```python
from build123d import *

# Parameters (mm, degrees)
F1_DEPTH = 25.4
F2_R     = 6.35
F3_DEPTH = 25.401
F4_DEPTH = 19.05
F5_R     = 6.35
F6_DEPTH = 6.351


with BuildPart() as f1:
    # F0 (on Top) → F1 (new body)
    with BuildSketch(Plane.XY):
        with BuildLine():
            ThreePointArc((-11.9960894898, 7.8287454173), (-22.8140252531, 16.2307401146), (-25.7390544228, 29.6122741608))
            ThreePointArc((-25.7390544228, 29.6122741608), (-33.3767507176, 24.6782589704), (-41.673253936, 28.3994073062))
            ThreePointArc((-41.673253936, 28.3994073062), (-43.3440087931, 16.5245060033), (-51.6016386333, 7.8287454173))
            ThreePointArc((-51.6016386333, 7.8287454173), (-44.8664465425, 5.0389375081), (-42.0766386333, -1.6962545827))
            ThreePointArc((-42.0766386333, -1.6962545827), (-43.013362785, -5.8153737791), (-45.6392933218, -9.1243137765))
            ThreePointArc((-45.6392933218, -9.1243137765), (-31.7988640615, -7.20255554), (-17.9584348012, -9.1243137765))
            ThreePointArc((-17.9584348012, -9.1243137765), (-20.9815746971, 1.463916392), (-11.9960894898, 7.8287454173))
        make_face()
        with BuildLine():
            ThreePointArc((-42.0766386333, -1.6962545827), (-44.8664465425, 5.0389375081), (-51.6016386333, 7.8287454173))
            ThreePointArc((-51.6016386333, 7.8287454173), (-61.1266386333, -1.6962545827), (-51.6016386333, -11.2212545827))
            ThreePointArc((-51.6016386333, -11.2212545827), (-48.6531092599, -10.0799677677), (-45.6392933218, -9.1243137765))
            ThreePointArc((-45.6392933218, -9.1243137765), (-43.013362785, -5.8153737791), (-42.0766386333, -1.6962545827))
        make_face()
        with BuildLine():
            ThreePointArc((-2.4710894898, -1.6962545827), (-5.260897399, 5.0389375081), (-11.9960894898, 7.8287454173))
            ThreePointArc((-11.9960894898, 7.8287454173), (-20.9815746971, 1.463916392), (-17.9584348012, -9.1243137765))
            ThreePointArc((-17.9584348012, -9.1243137765), (-14.9446188632, -10.0799677677), (-11.9960894898, -11.2212545827))
            ThreePointArc((-11.9960894898, -11.2212545827), (-5.260897399, -8.4314466735), (-2.4710894898, -1.6962545827))
        make_face()
        with BuildLine():
            ThreePointArc((-25.7390544228, 29.6122741608), (-25.2909601874, 31.9282439717), (-24.5746759409, 34.175785181))
            ThreePointArc((-24.5746759409, 34.175785181), (-34.0996759409, 43.700785181), (-43.6246759409, 34.175785181))
            ThreePointArc((-43.6246759409, 34.175785181), (-42.4236958583, 31.3636984394), (-41.673253936, 28.3994073062))
            ThreePointArc((-41.673253936, 28.3994073062), (-33.3767507176, 24.6782589704), (-25.7390544228, 29.6122741608))
        make_face()
    extrude(amount=F1_DEPTH)

    # F2 (on face) → F3 (cut, through all)
    with BuildSketch(Plane.XY.offset(25.4)):
        with Locations((-51.6016386333, -1.6962545827)):
            Circle(F2_R)
        with Locations((-11.9960894898, -1.6962545827)):
            Circle(F2_R)
        with Locations((-34.0996759409, 34.175785181)):
            Circle(F2_R)
    extrude(amount=-F3_DEPTH, mode=Mode.SUBTRACT)

    # F4 (cut): a face of the model
    f4_faces = [f1.faces().sort_by_distance(p)[0] for p in [
        (-32.4383450301, 9.0422986836, 25.4),
    ]]
    extrude(f4_faces, amount=-F4_DEPTH, mode=Mode.SUBTRACT)

    # F5 (on face) → F6 (cut, through all)
    with BuildSketch(Plane.XY.offset(6.35)):
        with Locations((-31.778564126, 13.1174343201)):
            Circle(F5_R)
    extrude(amount=-F6_DEPTH, mode=Mode.SUBTRACT)


solid = f1.part
```
Geometry check sheet. Reference: the model listing, model coordinates, mm. Give positions to 0.01 mm unless a question says otherwise; leave off trailing zeros. Write each loop counter-clockwise with the first axis right and the second up, starting at its lowest first coordinate (ties: lowest second). Pieces come first, ordered by that corner, then holes.
1) Section check D-D, the plane z = 4. Record the boundary of the cut face in (x, y) (3 decimals), and give its area (3 significant figures).
2) Gauge pin test, flat ends, axial feed: pin 1 (2 mm diameter, centred on y = 8, z = 3, fed in from +X); pin 2 (3 mm diameter, centred on x = -18.5, z = 4, fed in from +Y). Record the tip position at first contact, or that the pin passes through.
3) Material ranges on L1, parallel to Y at x = -31, z = 1; L2, parallel to Y at x = -29, z = 0.5; L3, parallel to X at y = 30, z = 1.75, recorded low to high.
4) Release check for a two-part mould opening along Y. For faces 1 (the cylindrical face through (-45.736, -4.128, 3.219)), 2 (the cylindrical face through (-61.124, -1.487, 3.131)), 3 (the cylindrical face through (-33.9, 43.7, 3.1)) record: pulls with the +Y half, pulls with the -Y half, needs draft (parallel to the pull), parting line crosses it, or undercut.
5) Section check B-B, the plane x = -50. Record the boundary of the cut face in (y, z).
6) Section check A-A, the plane y = -6.5. Record the boundary of the cut face in (x, z).
7) Section check C-C, the plane y = 33. Record the boundary of the cut face in (x, z).
Computed:
1. outline: (-51.602, -11.221) arc R50.8 cw to (-11.996, -11.221) arc R9.525 ccw to (-11.996, 7.829) arc R20.104 cw to (-24.575, 34.176) arc R9.525 ccw to (-43.625, 34.176) arc R19.662 cw to (-51.602, 7.829) arc R9.525 ccw to start; hole circle Ø12.7 at (-51.602, -1.696); hole circle Ø12.7 at (-34.1, 34.176); hole circle Ø12.7 at (-31.779, 13.117); hole circle Ø12.7 at (-11.996, -1.696)
1. area: 1,110 mm2
2. pin 1: stops at x = -8.11
2. pin 2: stops at y = 12.72
3. L1: y = -7.21 to 6.82, 19.42 to 28.63, 39.72 to 43.18
3. L2: y = -7.28 to 7.41, 18.83 to 30.39, 37.96 to 42.22
3. L3: x = -42.02 to -38.88, -29.32 to -25.68
4. face 1: undercut
4. face 2: parting line crosses it
4. face 3: pulls with the +Y half
5. outline: (-10.58, 0) - (-7.84, 0) - (-7.84, 6.35) - (-10.58, 6.35) - close; (4.45, 0) - (8.81, 0) - (8.81, 6.35) - (4.45, 6.35) - close
6. outline: (-59.83, 0) - (-55.75, 0) - (-55.75, 6.35) - (-59.83, 6.35) - close; (-47.45, 0) - (-16.15, 0) - (-16.15, 6.35) - (-47.45, 6.35) - close; (-7.84, 0) - (-3.77, 0) - (-3.77, 6.35) - (-7.84, 6.35) - close
7. outline: (-43.06, 0) - (-40.34, 0) - (-40.34, 6.35) - (-43.06, 6.35) - close; (-27.86, 0) - (-24.99, 0) - (-24.99, 6.35) - (-27.86, 6.35) - close
